from build123d import *

# Parameters (mm, degrees)
F0_W          = 50
F0_H          = 50
F1_DEPTH      = 1.62
F3_DEPTH      = 17
F2_W          = 20
F2_H          = 10.3
F4_DEPTH      = 14.3
F2_W_2        = 2.5
F2_H_2        = 5
F2_W_3        = 0.67
F2_H_3        = 0.67
F5_DEPTH      = 3
F6_DEPTH      = 8.5
F7_D          = 3.3
F9_DEPTH      = 18.84
F9_DEPTH_BACK = 13.66
F11_DEPTH     = 20


with BuildPart() as f1:
    # F0 (on Top) → F1 (new body)
    with BuildSketch(Plane.XY):
        Rectangle(F0_W, F0_H)
    extrude(amount=F1_DEPTH)

    # F2 (on face) → F3 (join)
    with BuildSketch(Plane.XY.offset(1.62)):
        with BuildLine():
            ThreePointArc((-6, 20), (-7.464466, 23.535534), (-11, 25))
            ThreePointArc((-11, 25), (-14.535534, 16.464466), (-6, 20))
        make_face()
    extrude(amount=F3_DEPTH)

    # F2 (on face) → F4 (join)
    with BuildSketch(Plane.XY.offset(1.62)):
        with Locations((4.576447, 19.85)):
            Rectangle(F2_W, F2_H)
    extrude(amount=F4_DEPTH)

    # F2 (on face) → F5 (join)
    with BuildSketch(Plane.XY.offset(1.62)):
        with Locations((13.75, -21.83)):
            Rectangle(F2_W_2, F2_H_2)
        with Locations((13.75, -23.08)):
            Rectangle(F2_W_3, F2_H_3, mode=Mode.SUBTRACT)
        with Locations((13.75, -20.58)):
            Rectangle(F2_W_3, F2_H_3, mode=Mode.SUBTRACT)
        with Locations((11.25, -21.83)):
            Rectangle(F2_W_2, F2_H_2)
        with Locations((11.25, -23.08)):
            Rectangle(F2_W_3, F2_H_3, mode=Mode.SUBTRACT)
        with Locations((11.25, -20.58)):
            Rectangle(F2_W_3, F2_H_3, mode=Mode.SUBTRACT)
        with Locations((8.75, -21.83)):
            Rectangle(F2_W_2, F2_H_2)
        with Locations((8.75, -23.08)):
            Rectangle(F2_W_3, F2_H_3, mode=Mode.SUBTRACT)
        with Locations((8.75, -20.58)):
            Rectangle(F2_W_3, F2_H_3, mode=Mode.SUBTRACT)
        with Locations((6.25, -21.83)):
            Rectangle(F2_W_2, F2_H_2)
        with Locations((6.25, -23.08)):
            Rectangle(F2_W_3, F2_H_3, mode=Mode.SUBTRACT)
        with Locations((6.25, -20.58)):
            Rectangle(F2_W_3, F2_H_3, mode=Mode.SUBTRACT)
    extrude(amount=F5_DEPTH)

    # F2 (on face) → F6 (join)
    with BuildSketch(Plane.XY.offset(1.62)):
        with Locations((6.25, -20.58)):
            Rectangle(F2_W_3, F2_H_3)
        with Locations((6.25, -23.08)):
            Rectangle(F2_W_3, F2_H_3)
        with Locations((8.75, -23.08)):
            Rectangle(F2_W_3, F2_H_3)
        with Locations((8.75, -20.58)):
            Rectangle(F2_W_3, F2_H_3)
        with Locations((11.25, -20.58)):
            Rectangle(F2_W_3, F2_H_3)
        with Locations((11.25, -23.08)):
            Rectangle(F2_W_3, F2_H_3)
        with Locations((13.75, -23.08)):
            Rectangle(F2_W_3, F2_H_3)
        with Locations((13.75, -20.58)):
            Rectangle(F2_W_3, F2_H_3)
    extrude(amount=F6_DEPTH)

    # F7 (through all)
    with Locations(Plane.XY.offset(1.62)):
        with Locations((-20, 18.5), (-20, -21.5), (20, -21.5), (20, 18.5)):
            Hole(F7_D / 2)

    # F8 (on Front) → F9 (join, two sides)
    with BuildSketch(Plane.XZ) as f9_sk:
        Polygon((25.5, -23.23), (25.5, 0), (-25.5, 0), (-25.5, -23.23), (-23.699168, -23.23), (-22.864854, -4.496027), (-21.367718, -4.496027), (-19.342193, -23.23), (-17.799168, -23.23), (-16.964854, -4.496027), (-15.467718, -4.496027), (-13.442193, -23.23), (-11.899168, -23.23), (-11.064854, -4.496027), (-9.567718, -4.496027), (-7.542193, -23.23), (-5.999168, -23.23), (-5.164854, -4.496027), (-3.667718, -4.496027), (-1.642193, -23.23), (-0.099168, -23.23), (0.735146, -4.496027), (2.232282, -4.496027), (4.257807, -23.23), (5.800832, -23.23), (6.635146, -4.496027), (8.132282, -4.496027), (10.157807, -23.23), (11.700832, -23.23), (12.535146, -4.496027), (14.032282, -4.496027), (16.057807, -23.23), (17.600832, -23.23), (18.435146, -4.496027), (19.932282, -4.496027), (21.957807, -23.23), align=None)
    extrude(amount=F9_DEPTH)
    extrude(f9_sk.sketch, amount=-F9_DEPTH_BACK)

    # F10 (on face) → F11 (cut)
    with BuildSketch(Plane.YZ.offset(14.576447)):
        Polygon((14.7, 15.92), (14.7, 6.684894), (18.009929, 15.92), align=None)
        Polygon((25, 15.92), (23.284927, 15.92), (24.399363, 9.693871), (25, 9.693871), align=None)
    extrude(amount=-F11_DEPTH, mode=Mode.SUBTRACT)


solid = f1.part
Work out the finished part from the listing and answer in its coordinate system (mm). A direction names the side the tool comes from. Give positions to 0.01 mm unless a question says otherwise; leave off trailing zeros. Loops run counter-clockwise (first coordinate to the right, second up) from the corner with the lowest first, then second, coordinate; pieces in that order, holes last. Notation, with made-up numbers: (-16, -3.75) -> (-8, -3.75) arc R21 cw to (-8, 16.25) -> close; hole circle Ø2 at (-31, 16). An arc over 180 degrees is marked (long way). Use a Markdown table: item, result. Add a question column.
1) The part is cut by section B-B, the plane z = 8. Count the separate pieces of the cut face and the enclosed holes in it, plus the area to 3 significant figures.
2) Which of the six approach directions +Z, -Z, +X, -X, +Y, -Y give full straight-line access (tool end or side, diameter ignored) to faces 4 (the flat face through (-25, 0, 1)), 5 (the flat face through (3.23, -2.82, -13.73)), 6 (the flat face through (0, -22, 0))?
3) For a pull along Y with two mould halves and no side action, classify faces 1 (the flat face through (10, -22, 4.62)), 2 (the flat face through (17, -3, -23.23)), 3 (the flat face through (10, -24.33, 3)) as +Y half, -Y half, draft (parallel to the pull), parting line (faces both ways), or undercut.
4) Each of these flat-tipped pins is pushed along its axis until it touches: P1, Ø0.7, axis at x = 9, y = -23, coming from the +Z side; P2, Ø1, axis at x = 12, z = -11, coming from the -Y side; P3, Ø2.5, axis at x = 5, y = 20, coming from the +Z side; P4, Ø2, axis at y = 13.5, z = 7.5, coming from the +X side. Where does it stop, or does it pass through?
5) Consider line 1 along Y through (x, z) = (-20, 0.75); line 2 along X through (y, z) = (18, 1); line 3 along X through (y, z) = (19.5, 1). Determine where each line is inside the solid, lowest interval first.
6) The part is cut by section A-A, the plane x = -8.5. Determine the outline of the cut face in (y, z).
Reported:
| question | item | result |
|---|---|---|
| 1 | separate pieces | 10 |
| 1 | enclosed holes | 0 |
| 1 | area | 279 mm^2 |
| 2 | face 4 | +Z, -X, +Y, -Y |
| 2 | face 5 | -Z, +Y, -Y |
| 2 | face 6 | -Z, +X, -X, -Y |
| 3 | face 1 | undercut |
| 3 | face 2 | draft |
| 3 | face 3 | -Y half |
| 4 | P1 | stops at z = 10.12 |
| 4 | P2 | stops at y = -18.84 |
| 4 | P3 | stops at z = 15.92 |
| 4 | P4 | passes through |
| 5 | line 1 | y = -25 to -23.15, -19.85 to 16.85, 20.15 to 25 |
| 5 | line 2 | x = -25 to -21.57, -18.43 to 18.43, 21.57 to 25 |
| 5 | line 3 | x = -25 to -21.31, -18.69 to 18.69, 21.31 to 25 |
| 6 | outline | (-25, 0) -> (-18.84, 0) -> (-18.84, -14.37) -> (13.66, -14.37) -> (13.66, 0) -> (25, 0) -> (25, 1.62) -> (24.33, 1.62) -> (24.33, 18.62) -> (15.67, 18.62) -> (15.67, 1.62) -> (-25, 1.62) -> close |
